from build123d import *

# Parameters (mm, degrees)
SKIZZE1_W                                     = 38
SKIZZE1_H                                     = 48
GRUNDPLATTE_DEPTH                             = 1.5
SKIZZE2_R                                     = 1.8
FC_BOHRUNGEN_DEPTH                            = 1.5
SKIZZE3_W                                     = 26.5
SKIZZE3_H                                     = 21
AUSCHNITT_EMPF_NGER_DEPTH                     = 31.647185841
SKIZZE4_W                                     = 26.5
SKIZZE4_H                                     = 21
SKIZZE4_W_2                                   = 21.5
SKIZZE4_H_2                                   = 17
AUFLAGEEMPF_NGER_DEPTH                        = 0.5
VERRUNDUNG1_R                                 = 2
LANGLOCHKABELBINDER_DEPTH                     = 31.647185841
SKIZZE8_W                                     = 12
SKIZZE8_H                                     = 5.25
AUFSATZ_LINEAR_AUSTRAGEN7_DEPTH               = 1.5
SKIZZE10_W                                    = 29.5
SKIZZE10_H                                    = 24
SKIZZE10_W_2                                  = 26.5
SKIZZE10_H_2                                  = 21
HALTERAHMEN_EMPF_NGER_DEPTH                   = 3
DURCHBRUCH_EMPF_NGER_REACH                    = 48.41
SKIZZE11_W                                    = 7
SKIZZE11_H                                    = 1
VERST_RKUNG_KABELBINDER_DEPTH                 = 3
VERRUNDUNG_VERST_RKUNG_KABELBINDER_R          = 2
AUSSCHNITT_ANTENNENANSATZEMPF_NGER_DEPTH      = 45.286707938
AUSSCHNITT_ANTENNENANSATZEMPF_NGER_DEPTH_BACK = 45.286707938
SKIZZE13_W                                    = 3.5
SKIZZE13_H                                    = 1.8
LANGLOCH_REPARATUR_DEPTH                      = 36.168345142
SKIZZE15_W                                    = 3.5
SKIZZE15_H                                    = 1.5
SCHNITT_LINEAR_AUSTRAGEN8_DEPTH               = 35.983603302
SKIZZE16_W                                    = 4.5
SKIZZE16_H                                    = 5.5
SCHNITT_LINEAR_AUSTRAGEN9_DEPTH               = 2
SCHNITT_LINEAR_AUSTRAGEN10_DEPTH              = 36.008034792
VERRUNDUNG6_R                                 = 1
VERRUNDUNG7_R                                 = 1.5
VERRUNDUNG8_R                                 = 1
VERRUNDUNG4_R                                 = 2
VERRUNDUNG5_R                                 = 1.5


with BuildPart() as part:
    # Skizze1 → Grundplatte (new body)
    with BuildSketch(Plane(origin=(0, 0, 0), x_dir=(1, 0, 0), z_dir=(0, 1, 0))):
        Rectangle(SKIZZE1_W, SKIZZE1_H)
    extrude(amount=GRUNDPLATTE_DEPTH)

    # Skizze2 → FC-Bohrungen (cut)
    with BuildSketch(Plane(origin=(0, 1.5, 0), x_dir=(1, 0, 0), z_dir=(0, 1, 0))):
        with Locations(Location((-15.25, 15.25, 0), (0, 0, 270))):
            Circle(SKIZZE2_R)
        with Locations(Location((15.25, 15.25, 0), (0, 0, 270))):
            Circle(SKIZZE2_R)
        with Locations(Location((15.25, -15.25, 0), (0, 0, 270))):
            Circle(SKIZZE2_R)
        with Locations(Location((-15.25, -15.25, 0), (0, 0, 270))):
            Circle(SKIZZE2_R)
    extrude(amount=-FC_BOHRUNGEN_DEPTH, mode=Mode.SUBTRACT)

    # Skizze3 → Auschnitt Empfänger (cut, through all)
    with BuildSketch(Plane(origin=(0, 1.5, 0), x_dir=(1, 0, 0), z_dir=(0, 1, 0))):
        with Locations((2, 0)):
            Rectangle(SKIZZE3_W, SKIZZE3_H)
    extrude(amount=-AUSCHNITT_EMPF_NGER_DEPTH, mode=Mode.SUBTRACT)

    # Skizze4 → AuflageEMpfänger (add)
    with BuildSketch(Plane.XZ):
        with Locations((2, 0)):
            Rectangle(SKIZZE4_W, SKIZZE4_H)
        with Locations((1.5, 0)):
            Rectangle(SKIZZE4_W_2, SKIZZE4_H_2, mode=Mode.SUBTRACT)
    extrude(amount=-AUFLAGEEMPF_NGER_DEPTH)

    # Verrundung1
    verrundung1_edges = [part.edges().sort_by_distance(p)[0] for p in [
        (-9.25, 0.25, 8.5),
        (12.25, 0.25, 8.5),
        (12.25, 0.25, -8.5),
        (-9.25, 0.25, -8.5),
    ]]
    fillet(verrundung1_edges, radius=VERRUNDUNG1_R)

    # Skizze7 → LanglochKabelbinder (cut, through all)
    with BuildSketch(Plane(origin=(0, 1.5, 0), x_dir=(1, 0, 0), z_dir=(0, 1, 0))):
        with BuildLine():
            Line((-9.25, 22.25), (-5.25, 22.25))
            ThreePointArc((-5.25, 22.25), (-4.5, 21.5), (-5.25, 20.75))
            Line((-5.25, 20.75), (-9.25, 20.75))
            ThreePointArc((-9.25, 20.75), (-10, 21.5), (-9.25, 22.25))
        make_face()
        with BuildLine():
            Line((-5.25, -22.25), (-9.25, -22.25))
            ThreePointArc((-9.25, -22.25), (-10, -21.5), (-9.25, -20.75))
            Line((-9.25, -20.75), (-5.25, -20.75))
            ThreePointArc((-5.25, -20.75), (-4.5, -21.5), (-5.25, -22.25))
        make_face()
    extrude(amount=-LANGLOCHKABELBINDER_DEPTH, mode=Mode.SUBTRACT)

    # Skizze8 → Aufsatz-Linear austragen7 (add, through all)
    with BuildSketch(Plane.XZ):
        with Locations((-7.25, 26.625)):
            Rectangle(SKIZZE8_W, SKIZZE8_H)
        with Locations((-7.25, -26.625)):
            Rectangle(SKIZZE8_W, SKIZZE8_H)
    extrude(amount=-AUFSATZ_LINEAR_AUSTRAGEN7_DEPTH)

    # Skizze10 → Halterahmen Empfänger (add)
    with BuildSketch(Plane(origin=(0, 1.5, 0), x_dir=(1, 0, 0), z_dir=(0, 1, 0))):
        with Locations((2, 0)):
            Rectangle(SKIZZE10_W, SKIZZE10_H)
        with Locations((2, 0)):
            Rectangle(SKIZZE10_W_2, SKIZZE10_H_2, mode=Mode.SUBTRACT)
    extrude(amount=HALTERAHMEN_EMPF_NGER_DEPTH)

    # Skizze11 → Durchbruch Empfänger (cut, up to next)
    with BuildSketch(Plane(origin=(16.75, 0, 0), x_dir=(0, 0, -1), z_dir=(1, 0, 0)), mode=Mode.PRIVATE) as durchbruch_empf_nger_sk1:
        with Locations((4, 4)):
            Rectangle(SKIZZE11_W, SKIZZE11_H)
    durchbruch_empf_nger_tool1 = extrude(durchbruch_empf_nger_sk1.sketch, amount=-DURCHBRUCH_EMPF_NGER_REACH, mode=Mode.PRIVATE) & part.part
    add(durchbruch_empf_nger_tool1.solids().sort_by_distance((16.75, 4, -4))[0], mode=Mode.SUBTRACT)

    # Skizze12 → Verstärkung Kabelbinder (add)
    with BuildSketch(Plane(origin=(0, 1.5, 0), x_dir=(1, 0, 0), z_dir=(0, 1, 0))):
        Polygon((-13.25, -24), (-13.25, -29.25), (-1.25, -29.25), (-1.25, -24), (-4.25, -12), (-10.25, -12), align=None)
        Polygon((-10.25, 12), (-13.25, 24), (-13.25, 29.25), (-1.25, 29.25), (-1.25, 24), (-4.25, 12), align=None)
    extrude(amount=VERST_RKUNG_KABELBINDER_DEPTH)

    # Verrundung Verstärkung Kabelbinder
    # the kernel refuses this fillet: 2 mm, written as the material it adds along each edge
    with BuildSketch(Plane(origin=(-4.25, 1.5, -12), x_dir=(0.2425356250363328, 0, -0.9701425001453319), z_dir=(0, 1, 0)), Plane(origin=(-4.25, 1.5, 12), x_dir=(1, 0, 0), z_dir=(0, 1, 0))) as verrundung_verst_rkung_kabelbinder_piece_1:
        with BuildLine():
            CenterArc((VERRUNDUNG_VERST_RKUNG_KABELBINDER_R * 1.2807764064, -VERRUNDUNG_VERST_RKUNG_KABELBINDER_R), VERRUNDUNG_VERST_RKUNG_KABELBINDER_R, 90, 104.036243468)
            Line((VERRUNDUNG_VERST_RKUNG_KABELBINDER_R * 0.310633906259, -VERRUNDUNG_VERST_RKUNG_KABELBINDER_R * 1.24253562504), (0, 0))
            Line((0, 0), (VERRUNDUNG_VERST_RKUNG_KABELBINDER_R * 1.2807764064, 0))
        make_face()
    extrude(amount=3)
    with BuildSketch(Plane(origin=(-10.25, 1.5, -12), x_dir=(-1, 0, 0), z_dir=(0, 1, 0))) as verrundung_verst_rkung_kabelbinder_piece_2_section:
        with BuildLine():
            CenterArc((VERRUNDUNG_VERST_RKUNG_KABELBINDER_R * 1.2807764064, -VERRUNDUNG_VERST_RKUNG_KABELBINDER_R), VERRUNDUNG_VERST_RKUNG_KABELBINDER_R, 90, 104.036243468)
            Line((VERRUNDUNG_VERST_RKUNG_KABELBINDER_R * 0.310633906259, -VERRUNDUNG_VERST_RKUNG_KABELBINDER_R * 1.24253562504), (0, 0))
            Line((0, 0), (VERRUNDUNG_VERST_RKUNG_KABELBINDER_R * 1.2807764064, 0))
        make_face()
    verrundung_verst_rkung_kabelbinder_piece_2 = extrude(amount=3, mode=Mode.PRIVATE)
    verrundung_verst_rkung_kabelbinder_piece_2 = split(verrundung_verst_rkung_kabelbinder_piece_2, bisect_by=Plane(origin=(-12.75, 3, -12.581943017), z_dir=(1, 0, 0)), keep=Keep.TOP, mode=Mode.PRIVATE)
    add(verrundung_verst_rkung_kabelbinder_piece_2)
    with BuildSketch(Plane(origin=(-10.25, 1.5, 12), x_dir=(-1, 0, 0), z_dir=(0, 1, 0))) as verrundung_verst_rkung_kabelbinder_piece_3_section:
        with BuildLine():
            CenterArc((VERRUNDUNG_VERST_RKUNG_KABELBINDER_R * 1.2807764064, VERRUNDUNG_VERST_RKUNG_KABELBINDER_R), VERRUNDUNG_VERST_RKUNG_KABELBINDER_R, 165.963756532, 104.036243468)
            Line((VERRUNDUNG_VERST_RKUNG_KABELBINDER_R * 0.310633906259, VERRUNDUNG_VERST_RKUNG_KABELBINDER_R * 1.24253562504), (0, 0))
            Line((0, 0), (VERRUNDUNG_VERST_RKUNG_KABELBINDER_R * 1.2807764064, 0))
        make_face()
    verrundung_verst_rkung_kabelbinder_piece_3 = extrude(amount=3, mode=Mode.PRIVATE)
    verrundung_verst_rkung_kabelbinder_piece_3 = split(verrundung_verst_rkung_kabelbinder_piece_3, bisect_by=Plane(origin=(-12.75, 3, 12.581943017), z_dir=(1, 0, 0)), keep=Keep.TOP, mode=Mode.PRIVATE)
    add(verrundung_verst_rkung_kabelbinder_piece_3)

    # Skizze13 → Ausschnitt AntennenAnsatzEmpfänger (cut, two sides: drawn at the far end of the back side and taken through both)
    with BuildSketch(Plane.XY.offset(-10.5).offset(-AUSSCHNITT_ANTENNENANSATZEMPF_NGER_DEPTH_BACK)):
        with Locations((-7.25, 3.6)):
            Rectangle(SKIZZE13_W, SKIZZE13_H)
    extrude(amount=AUSSCHNITT_ANTENNENANSATZEMPF_NGER_DEPTH + AUSSCHNITT_ANTENNENANSATZEMPF_NGER_DEPTH_BACK, mode=Mode.SUBTRACT)

    # Skizze14 → Langloch Reparatur (cut, through all)
    with BuildSketch(Plane.XZ):
        with BuildLine():
            Line((-5.25, 20.75), (-9.25, 20.75))
            ThreePointArc((-9.25, 20.75), (-10, 21.5), (-9.25, 22.25))
            Line((-9.25, 22.25), (-5.25, 22.25))
            ThreePointArc((-5.25, 22.25), (-4.5, 21.5), (-5.25, 20.75))
        make_face()
        with BuildLine():
            Line((-5.25, -22.25), (-9.25, -22.25))
            ThreePointArc((-9.25, -22.25), (-10, -21.5), (-9.25, -20.75))
            Line((-9.25, -20.75), (-5.25, -20.75))
            ThreePointArc((-5.25, -20.75), (-4.5, -21.5), (-5.25, -22.25))
        make_face()
    extrude(amount=-LANGLOCH_REPARATUR_DEPTH, mode=Mode.SUBTRACT)

    # Skizze15 → Schnitt-Linear austragen8 (cut, through all)
    with BuildSketch(Plane(origin=(0, 2.7, 0), x_dir=(1, 0, 0), z_dir=(0, 1, 0))):
        with Locations((-7.25, 28.5)):
            Rectangle(SKIZZE15_W, SKIZZE15_H)
        with Locations((-7.25, -28.5)):
            Rectangle(SKIZZE15_W, SKIZZE15_H)
    extrude(amount=-SCHNITT_LINEAR_AUSTRAGEN8_DEPTH, mode=Mode.SUBTRACT)

    # Skizze16 → Schnitt-Linear austragen9 (cut)
    with BuildSketch(Plane(origin=(0, 4.5, 0), x_dir=(1, 0, 0), z_dir=(0, 1, 0))):
        with Locations((-7.25, 21.5)):
            Rectangle(SKIZZE16_W, SKIZZE16_H)
        with Locations((-7.25, -21.5)):
            Rectangle(SKIZZE16_W, SKIZZE16_H)
    extrude(amount=-SCHNITT_LINEAR_AUSTRAGEN9_DEPTH, mode=Mode.SUBTRACT)

    # Skizze17 → Schnitt-Linear austragen10 (cut, through all)
    with BuildSketch(Plane(origin=(0, 1.5, 0), x_dir=(1, 0, 0), z_dir=(0, 1, 0))):
        Polygon((16.75, 12), (19, 13.88797417), (19, -13.88797417), (16.75, -12), align=None)
        Polygon((-12.75, 7.5), (-19, 12.744372695), (-19, -12.744372695), (-12.75, -7.5), align=None)
        Polygon((-19, 18.25), (-13.25, 24), (-19, 24), align=None)
        Polygon((-1.25, 24), (3.039498988, 18.88797417), (19, 18.88797417), (19, 24), align=None)
        Polygon((-19, -24), (-19, -18.25), (-13.25, -24), align=None)
        Polygon((19, -24), (-1.25, -24), (3.039498988, -18.88797417), (19, -18.88797417), align=None)
    extrude(amount=-SCHNITT_LINEAR_AUSTRAGEN10_DEPTH, mode=Mode.SUBTRACT)

    # Verrundung6
    verrundung6_edges = [part.edges().sort_by_distance(p)[0] for p in [
        (-7.25, 2.7, -27.75),
        (-7.25, 2.7, 27.75),
    ]]
    fillet(verrundung6_edges, radius=VERRUNDUNG6_R)

    # Verrundung7
    verrundung7_edges = [part.edges().sort_by_distance(p)[0] for p in [
        (16.75, 0.75, 12),
        (16.75, 0.75, -12),
        (19, 0.75, -13.88797417),
        (19, 0.75, 13.88797417),
        (-12.75, 0.75, -7.5),
        (-12.75, 0.75, 7.5),
        (-19, 0.75, 12.744372695),
        (-19, 0.75, -12.744372695),
    ]]
    fillet(verrundung7_edges, radius=VERRUNDUNG7_R)

    # Verrundung8
    verrundung8_edges = [part.edges().sort_by_distance(p)[0] for p in [
        (-5.5, 2.7, 14.625),
        (-9, 2.7, 14.625),
        (-5.5, 2.7, -14.625),
        (-9, 2.7, -14.625),
    ]]
    fillet(verrundung8_edges, radius=VERRUNDUNG8_R)

    # Verrundung4
    verrundung4_edges = [part.edges().sort_by_distance(p)[0] for p in [
        (-13.25, 2.25, 29.25),
        (-1.25, 2.25, 29.25),
        (-1.25, 2.25, -29.25),
        (-13.25, 2.25, -29.25),
        (-13.25, 0.75, -24),
        (-19, 0.75, -18.25),
        (-1.25, 0.75, -24),
        (3.039498988, 0.75, -18.88797417),
        (19, 0.75, -18.88797417),
        (19, 0.75, 18.88797417),
        (3.039498988, 0.75, 18.88797417),
        (-1.25, 0.75, 24),
        (-19, 0.75, 18.25),
        (-13.25, 0.75, 24),
    ]]
    fillet(verrundung4_edges, radius=VERRUNDUNG4_R)

    # Verrundung5
    verrundung5_edges = [part.edges().sort_by_distance(p)[0] for p in [
        (-12.75, 3, -12.000947412),
        (-12.75, 3, 12.000947412),
    ]]
    fillet(verrundung5_edges, radius=VERRUNDUNG5_R)


solid = part.part
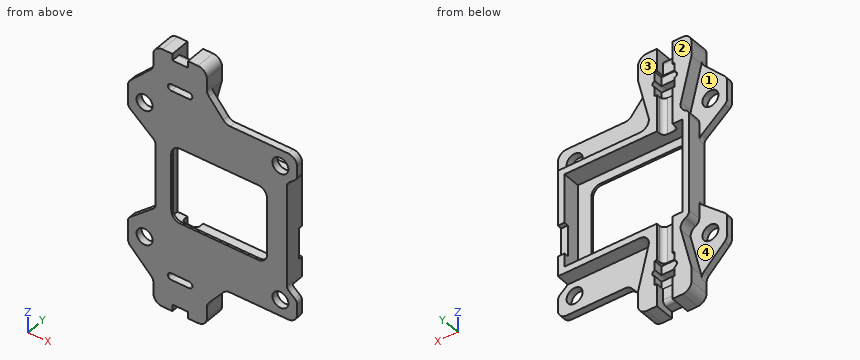
For this review, take the finished solid that the model builds, in its own axes (mm). Face numbers are marked on the shaded views. A direction names the side the tool comes from. Round coordinates to 2 decimals unless told otherwise and drop trailing zeros. Order: outer loops, then holes, each group sorted by start corner. A loop starts at its lowest first (then second) coordinate and runs counter-clockwise, first axis right, second up. Notation, with made-up numbers: M 69,73 L 103,73 A28 ccw 103,104 Z; hole C 21,28.5 d9. An arc over 180 degrees is marked long. Use a Markdown table: item, result. Add a question column.
Item 1: Add section C-C, the plane z = -15.25. Give the boundary of the cut face in (x, y), then the cut area to 3 significant figures.
Item 2: To check wall thickness, follow line 1 along X through (y, z) = (1.1, 15.25); line 2 along Z through (x, y) = (-8.5, 1.95); line 3 along X through (y, z) = (3.65, 5.5). State the ranges of each line that lie inside material, in increasing order.
Item 3: Add section A-A, the plane x = 7. Give the boundary of the cut face in (y, z).
Item 4: Add section D-D, the plane z = -21.5. Give the boundary of the cut face in (x, y) (3 decimals).
Item 5: Mouldability with a two-part tool opening along Z and no side actions: class the marked faces 3 and 4 as released by +Z, released by -Z, zero draft, split by the parting line, or undercut.
Item 6: Add section B-B, the plane z = 5. Give the boundary of the cut face in (x, y), then the cut area to 3 significant figures.
Item 7: Insertion check: pin 1 (0.6 mm diameter, centred on y = 3.5, z = 23, fed in from +X) (3 decimals); pin 2 (1.2 mm diameter, centred on x = 16, z = -5, fed in from +Y); pin 3 (1 mm diameter, centred on y = 3, z = -19.5, fed in from +X). Each pin has a flat end and moves straight along its axis. Give the tip position at first contact, or say it passes through.
Item 8: Tool access review of the marked faces 1 and 2: name each direction out of +Z, -Z, +X, -X, +Y, -Y from which nothing blocks a thin tool from reaching the whole face with its end or side.
Geometry results:
| question | item | result |
|---|---|---|
| 1 | outline | M -19,0 L -17.05,0 L -17.05,1.5 L -19,1.5 Z; M -13.45,0 L 13.45,0 L 13.45,1.5 L -3.44,1.5 L -3.44,4.5 L -5.5,4.5 L -5.5,3.7 A1 cw -6.5,2.7 L -8,2.7 A1 cw -9,3.7 L -9,4.5 L -11.06,4.5 L -11.06,1.5 L -13.45,1.5 Z; M 17.05,0 L 19,0 L 19,1.5 L 17.05,1.5 Z |
| 1 | area | 63.2 mm² |
| 2 | line 1 | x = -19 to -17.05, -13.45 to 13.45, 17.05 to 19 |
| 2 | line 2 | z = -27.72 to -22.25, -20.75 to -10.5, 10.5 to 20.75, 22.25 to 27.72 |
| 2 | line 3 | x = -12.75 to -11.25, 15.25 to 16.75 |
| 3 | outline | M 0,-18.89 L 1.5,-18.89 L 1.5,-12 L 4.5,-12 L 4.5,-10.5 L 0.5,-10.5 L 0.5,-8.5 L 0,-8.5 Z; M 0,8.5 L 0.5,8.5 L 0.5,10.5 L 4.5,10.5 L 4.5,12 L 1.5,12 L 1.5,18.89 L 0,18.89 Z |
| 4 | outline | M -15.75,0 L -10,0 L -10,4.5 L -12.625,4.5 L -12.625,1.5 L -15.75,1.5 Z; M -4.5,0 L 0.848,0 L 0.848,1.5 L -1.875,1.5 L -1.875,4.5 L -4.5,4.5 Z |
| 5 | face 3 | zero draft |
| 5 | face 4 | undercut |
| 6 | outline | M -12.75,0 L -9.25,0 L -9.25,0.5 L -11.25,0.5 L -11.25,4.5 L -12.75,4.5 Z; M 12.25,0 L 16.75,0 L 16.75,4.5 L 15.25,4.5 L 15.25,0.5 L 12.25,0.5 Z |
| 6 | area | 16.0 mm² |
| 7 | pin 1 | stops at x = -1.425 |
| 7 | pin 2 | stops at y = 3.5 |
| 7 | pin 3 | stops at x = -2.25 |
| 8 | face 1 | -X, +Y |
| 8 | face 2 | +Z, -Z, +X, -X, +Y |
